Read the model definition and answer for the solid it produces. Units are mm, in the model's axes. Face numbers are marked on the shaded views. Round coordinates to 2 decimals unless told otherwise and drop trailing zeros. Order: outer loops, then holes, each group sorted by start corner. A loop starts at its lowest first (then second) coordinate and runs counter-clockwise, first axis right, second up. Notation, with made-up numbers: M -4.5,26 L 36.5,26 A21 cw 36.5,51 Z; hole C 82.25,61.5 d7. An arc over 180 degrees is marked long. Use one line per item in the form item = value. Start each with the question number.
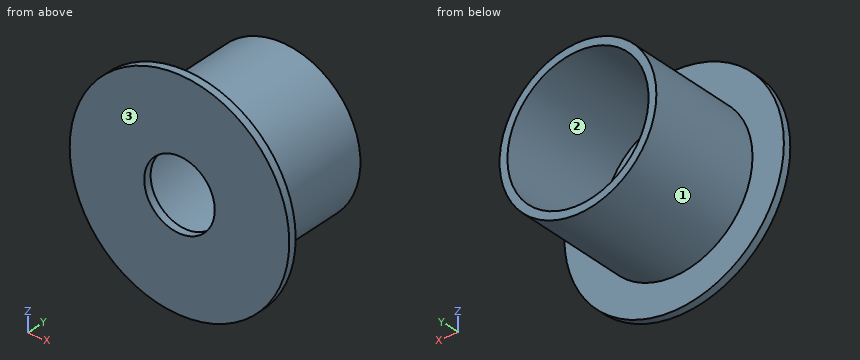
Autodesk Inventor part; units mm, degrees
ref_plane "YZ Plane" through (0, 0, 0) normal (1, 0, 0) x (0, 1, 0)
ref_plane "XZ Plane" through (0, 0, 0) normal (0, 1, 0) x (-1, 0, 0)
ref_plane "XY Plane" through (0, 0, 0) normal (0, 0, 1) x (1, 0, 0)
sketch "Szkic1" plane through (0, 0, 0) normal (0, 1, 0) x (-1, 0, 0)
  circle A0 centre (0, 0) radius 50
  dimension "d0" = 100
extrude "Wyciągnięcie proste1" add sketch "Szkic1" along normal blind 80
sketch "Szkic2" plane through (0, 80, 0) normal (0, 1, 0) x (1, 0, 0)
  circle A0 centre (0, 0) radius 45
  dimension "d3" = 90
extrude "Wyciągnięcie proste2" cut sketch "Szkic2" against normal blind 75
sketch "Szkic3" plane through (0, 5, 0) normal (0, 1, 0) x (1, 0, 0)
  point P0 (0, 0)
sketch "Szkic4" plane through (0, 5, 0) normal (0, 1, 0) x (1, 0, 0)
  circle A0 centre (0, 0) radius 22.5
  dimension "d6" = 45
extrude "Wyciągnięcie proste3" cut sketch "Szkic4" against normal blind 75
sketch "Szkic9" plane through (0, 5, 0) normal (0, 1, 0) x (1, 0, 0)
  point P0 (0, 0)
sketch "Szkic10" plane through (0, 0, 0) normal (0, -1, 0) x (1, 0, 0)
  circle A0 centre (0, 0) radius 70
  circle A1 centre (0, 0) radius 40.2417
  dimension "d14" = 140
extrude "Wyciągnięcie proste4" add sketch "Szkic10" against normal blind 5
sketch "Szkic11" plane through (0, 5, 0) normal (0, 1, 0) x (1, 0, 0)
  point P0 (0, 0)
properties part number "Walec"
Item 1: Section A-A (z = 0) is taken. Write down the section's boundary in (x, y), and give its area (4 significant figures).
Item 2: Section D-D (z = 37) is taken. Write down the section's boundary in (x, y).
Item 3: Given P1, Ø5, axis at x = -27.5, z = 19.5, coming from the +Y side; P2, Ø5, axis at y = 45.5, z = -8.5, coming from the +X side; P3, Ø1, axis at y = 27.5, z = 15.5, coming from the -X side, each flat-ended and moving along its own axis, determine where each tip first touches the part or whether it passes through.
Item 4: For a pull along Z with two mould halves and no side action, classify the marked faces 1, 2 and 3 as pulls with the +Z half, pulls with the -Z half, needs draft (parallel to the pull), parting line crosses it, or undercut.
Item 5: Section C-C (y = 60) is taken. Write down the section's boundary in (x, z), and give its area (3 significant figures).
Item 6: Find the intervals of material crossed by L1, parallel to Z at x = 0, y = 3; L2, parallel to Z at x = 0.5, y = 63; L3, parallel to Y at x = 24.5, z = 21, in increasing order. Write a range as [from, to].
Item 7: Section B-B (x = 2.5) is taken. Write down the section's boundary in (y, z), and give its area (3 significant figures).
The answers:
q1.outline = M -70,0 L -22.5,0 L -22.5,5 L -45,5 L -45,80 L -50,80 L -50,5 L -70,5 Z; M 22.5,0 L 70,0 L 70,5 L 50,5 L 50,80 L 45,80 L 45,5 L 22.5,5 Z
q1.area = 1,225 mm²
q2.outline = M -59.42,0 L 59.42,0 L 59.42,5 L 33.63,5 L 33.63,80 L 25.61,80 L 25.61,5 L -25.61,5 L -25.61,80 L -33.63,80 L -33.63,5 L -59.42,5 Z
q3.P1 = 5
q3.P2 = 49.64
q3.P3 = -47.7
q4.face_1 = parting line crosses it
q4.face_2 = undercut
q4.face_3 = needs draft
q5.outline = C 0,0 d100; hole C 0,0 d90
q5.area = 1,490 mm²
q6.L1 = [-70, -22.5], [22.5, 70]
q6.L2 = [-50, -45], [45, 50]
q6.L3 = [0, 5]
q7.outline = M 0,-69.96 L 5,-69.96 L 5,-49.94 L 80,-49.94 L 80,-44.93 L 5,-44.93 L 5,-22.36 L 0,-22.36 Z; M 0,22.36 L 5,22.36 L 5,44.93 L 80,44.93 L 80,49.94 L 5,49.94 L 5,69.96 L 0,69.96 Z
q7.area = 1,230 mm²
